```python
from build123d import *

# Parameters (mm, degrees)
SKETCH1_W           = 40
SKETCH1_H           = 15
SKETCH1_R           = 2.25
SKETCH1_R_2         = 2.1
BOSS_EXTRUDE1_DEPTH = 2
SKETCH2_W           = 40
SKETCH2_H           = 2
BOSS_EXTRUDE2_DEPTH = 28
SKETCH3_W           = 40
SKETCH3_H           = 2
BOSS_EXTRUDE3_DEPTH = 20
SKETCH4_R           = 1.5
CUT_EXTRUDE1_DEPTH  = 20
FILLET1_R           = 1
BOSS_EXTRUDE4_START = 2
BOSS_EXTRUDE4_DEPTH = 2


with BuildPart() as part:
    # Sketch1 → Boss-Extrude1 (new body)
    with BuildSketch(Plane(origin=(0, 0, 0), x_dir=(1, 0, 0), z_dir=(0, 1, 0))):
        with Locations((20, 7.5)):
            Rectangle(SKETCH1_W, SKETCH1_H)
        with Locations(Location((15, 10.8, 0), (0, 0, 270))):
            Circle(SKETCH1_R, mode=Mode.SUBTRACT)
        with Locations(Location((25, 10.8, 0), (0, 0, 270))):
            Circle(SKETCH1_R_2, mode=Mode.SUBTRACT)
    extrude(amount=-BOSS_EXTRUDE1_DEPTH)

    # Sketch2 → Boss-Extrude2 (add)
    with BuildSketch(Plane.XZ.offset(2)):
        with Locations((20, -1)):
            Rectangle(SKETCH2_W, SKETCH2_H)
    extrude(amount=BOSS_EXTRUDE2_DEPTH)

    # Sketch3 → Boss-Extrude3 (add)
    with BuildSketch(Plane.XY):
        with Locations((20, -29)):
            Rectangle(SKETCH3_W, SKETCH3_H)
    extrude(amount=BOSS_EXTRUDE3_DEPTH)

    # Sketch4 → Cut-Extrude1 (cut)
    with BuildSketch(Plane(origin=(0, -28, 0), x_dir=(1, 0, 0), z_dir=(0, 1, 0))):
        with Locations(Location((10, -10, 0), (0, 0, 180))):
            Circle(SKETCH4_R)
        with Locations(Location((30, -10, 0), (0, 0, 180))):
            Circle(SKETCH4_R)
    extrude(amount=-CUT_EXTRUDE1_DEPTH, mode=Mode.SUBTRACT)

    # Fillet1
    fillet1_edges = [part.edges().sort_by_distance(p)[0] for p in [
        (20, -2, -2),
        (20, -30, -2),
        (20, -28, 0),
        (20, 0, 0),
    ]]
    fillet(fillet1_edges, radius=FILLET1_R)

    # Sketch5 → Boss-Extrude4 (add)
    with BuildSketch(Plane(origin=(0, 0, 0), x_dir=(0, 0, -1), z_dir=(1, 0, 0)).offset(BOSS_EXTRUDE4_START)):
        with BuildLine():
            Line((0, -18), (-10, -28))
            Line((-10, -28), (-1, -28))
            ThreePointArc((-1, -28), (-0.292893219, -27.707106781), (0, -27))
            Line((0, -27), (0, -18))
        make_face()
    boss_extrude4 = extrude(amount=-BOSS_EXTRUDE4_DEPTH)

    # Mirror1: Boss-Extrude4 across plane
    add(boss_extrude4.mirror(Plane(origin=(20, 0, 0), x_dir=(0, 0, 1), z_dir=(1, 0, 0))))


solid = part.part
```
Geometry: final body of the model. Coordinates: model frame, mm. A direction names the side the tool comes from. Round coordinates to 2 decimals unless told otherwise and drop trailing zeros. Order: outer loops, then holes, each group sorted by start corner. A loop starts at its lowest first (then second) coordinate and runs counter-clockwise, first axis right, second up. Notation, with made-up numbers: (47.5, -33.5) - (87.5, -33.5) arc R31 ccw to (87.5, -1.5) - close; hole circle Ø2 at (-7.75, 13.25). An arc over 180 degrees is marked (long way). Write item = value, one per line. Start each with the question number.
Q1. Pin query (flat end, axial travel): pin 1 (1.5 mm diameter, centred on y = -26.5, z = -4.5, fed in from -X); pin 2 (13 mm diameter, centred on x = 18, y = -14.5, fed in from +Z); pin 3 (5 mm diameter, centred on x = 30, z = 10, fed in from +Y); pin 4 (8 mm diameter, centred on x = 17, y = -17, fed in from -Z). Return the tip coordinate at first contact, or that it passes through.
Q2. Ray query, line 1 (X direction, y = -1.4, z = -10.8); line 2 (Z direction, x = 10, y = -28.55); line 3 (Y direction, x = 35, z = 1). Return the intervals inside material, ascending. Write a range as from..to.
Q3. Cut plane D-D on z = 13. Return the cut outline in (x, y), and give its area (3 significant figures).
Q4. Cut plane B-B on y = -23.25. Return the cut outline in (x, z), and give its area (3 significant figures).
Q5. Cut plane A-A on x = 30. Return the cut outline in (y, z), and give its area (3 significant figures).
Q6. Pull-direction query (X, two-part tool) for faces 4 (the cylindrical face through (12.804, -0.986, -11.288)), 5 (the flat face through (20, -30, 9)), 6 (the flat face through (40, -18.3, 0)); classes: +X half, -X half, draft (parallel to the pull), parting line (faces both ways), or undercut.
Q7. Cut plane C-C on x = 15. Return the cut outline in (y, z).
Q8. Access query for faces 1 (the cylindrical face through (20.252, -27.715, 0.301)), 2 (the flat face through (20, -2, -9)), 3 (the cylindrical face through (11.2, -29, 9.1)). Directions: +Z, -Z, +X, -X, +Y, -Y. A direction counts if a zero-diameter tool reaches every point of the face in a straight line with its end or side. Return the directions, or none.
Outcome:
q1.pin_1 = through
q1.pin_2 = 0
q1.pin_3 = -28
q1.pin_4 = -2
q2.line_1 = 0..12.75, 17.25..22.9, 27.1..40
q2.line_2 = -2..8.5, 11.5..20
q2.line_3 = -30..-28
q3.outline = (0, -30) - (40, -30) - (40, -28) - (0, -28) - close
q3.area = 80.0 mm^2
q4.outline = (0, -2) - (40, -2) - (40, 5.25) - (38, 5.25) - (38, 0) - (2, 0) - (2, 5.25) - (0, 5.25) - close
q4.area = 101 mm^2
q5.outline = (-30, -1) arc R1 ccw to (-29, -2) - (-3, -2) arc R1 cw to (-2, -3) - (-2, -15) - (0, -15) - (0, -1) arc R1 ccw to (-1, 0) - (-27, 0) arc R1 cw to (-28, 1) - (-28, 8.5) - (-30, 8.5) - close; (-30, 11.5) - (-28, 11.5) - (-28, 20) - (-30, 20) - close
q5.area = 120 mm^2
q6.face_4 = undercut
q6.face_5 = draft
q6.face_6 = +X half
q7.outline = (-30, -1) arc R1 ccw to (-29, -2) - (-3, -2) arc R1 cw to (-2, -3) - (-2, -8.55) - (0, -8.55) - (0, -1) arc R1 ccw to (-1, 0) - (-27, 0) arc R1 cw to (-28, 1) - (-28, 20) - (-30, 20) - close; (-2, -15) - (0, -15) - (0, -13.05) - (-2, -13.05) - close
q8.face_1 = +Z, +Y
q8.face_2 = -Z, +X, -X, -Y
q8.face_3 = +Y, -Y
